Geometry check sheet. Reference: the model listing, model coordinates, mm. A direction names the side the tool comes from. Round coordinates to 2 decimals unless told otherwise and drop trailing zeros. Write each loop counter-clockwise with the first axis right and the second up, starting at its lowest first coordinate (ties: lowest second). Pieces come first, ordered by that corner, then holes. Notation, with made-up numbers: M 68,-39.5 L 116,-39.5 A20 cw 116,-7.5 Z; hole C -24.5,28.25 d3. An arc over 180 degrees is marked long. Answer in a Markdown table with one row per item. Add a question column.
from build123d import *

# Parameters (mm, degrees)
F3_DEPTH        = 5.5
F5_D            = 3.6
F5_COPIES_COUNT = 3
F6_SIZE         = 0.3


# Not quite as in the source:
# - a pattern or mirror of a feature is missing from the dataset's text; its kind, count and spacing are read off the source's solid


with BuildPart() as f1:
    # F0 (on Front) → F1 (revolve)
    with BuildSketch(Plane.XZ):
        Polygon((0, 11), (0, 0), (42, 0), (44.5, 2.5), (52.5, 2.5), (52.5, 3.5), (12, 3.5), (12, 2.5), (10, 2.5), (10, 3.5), (2, 3.5), (2, 11), align=None)
    revolve(axis=Axis((21, 0, 0), (-1, 0, 0)))

    # F2 (on face) → F3 (cut)
    with BuildSketch(Plane.YZ.offset(52.5)):
        with BuildLine():
            Line((2.5, 0), (3.5, 0))
            ThreePointArc((3.5, 0), (0, 3.5), (-3.5, 0))
            Line((-3.5, 0), (-2.5, 0))
            ThreePointArc((-2.5, 0), (0, 2.5), (2.5, 0))
        make_face()
    extrude(amount=-F3_DEPTH, mode=Mode.SUBTRACT)

    # F5 (through all)
    with Locations(Plane(origin=(0, 0, 0), x_dir=(0, -1, 0), z_dir=(-1, 0, 0))):
        with Locations((0, 7)):
            f5 = Hole(F5_D / 2)

    # F5_copies: F5 ×3 about axis
    f5_copies_axis = Axis((0, 0, 0), (1, 0, 0))
    for i in range(1, F5_COPIES_COUNT):
        add(f5.rotate(f5_copies_axis, i * 360 / F5_COPIES_COUNT), mode=Mode.SUBTRACT)

    # F6
    f6_edges = [f1.edges().sort_by_distance(p)[0] for p in [
        (0, 0, -11),
        (0, -6.962178, -1.941154),
        (0, 5.162178, -5.058846),
        (0, 1.8, 7),
    ]]
    chamfer(f6_edges, length=F6_SIZE)


solid = f1.part
Item 1: Access from +Z, -Z, +X, -X, +Y, -Y to the whole of each face (thin tool, end or side, straight path). Record for faces 4 (the cylindrical face through (31.966, 0.154, -3.497)), 5 (the flat face through (47, 0, 3)), 6 (the flat face through (12, -2, 2)), 7 (the cylindrical face through (1.162, -0.39, 5.243)), 8 (the flat face through (52.5, 0, -3)).
Item 2: Section check A-A, the plane x = 29. Record the boundary of the cut face in (y, z).
Item 3: Gauge pin test, flat ends, axial feed: pin 1 Ø3 at (y, z) = (-6.06, -3.5) entering from +X; pin 2 Ø4 at (x, z) = (13, -2.5) entering from +Y; pin 3 Ø0.8 at (x, y) = (51, 3) entering from +Z; pin 4 Ø8 at (x, z) = (45, -3.5) entering from -Y. Record the tip position at first contact, or that the pin passes through.
Item 4: Mould release check, pull along Y, two halves, no side actions. Record for faces 1 (the cylindrical face through (10.99, -2.44, -0.54)), 2 (the flat face through (50, -3, 0)), 3 (the cylindrical face through (1.162, 7.725, -4.189)): +Y half, -Y half, draft (parallel to the pull), parting line (faces both ways), or undercut.
Item 5: Section check B-B, the plane x = 48. Record the boundary of the cut face in (y, z), and give its area (3 significant figures).
Item 6: Scan lines: probe 1 along X at (y, z) = (-7.25, 3.75); probe 2 along Z at (x, y) = (46.5, 0); probe 3 along Z at (x, y) = (21.5, 3). Record each from-to range of solid material in increasing order. Write a range as from..to.
Result sheet:
| question | item | result |
|---|---|---|
| 1 | face 4 | +X |
| 1 | face 5 | +Z, +X, +Y, -Y |
| 1 | face 6 | none |
| 1 | face 7 | +X, -X |
| 1 | face 8 | +Z, -Z, +X, +Y, -Y |
| 2 | outline | C 0,0 d7 |
| 3 | pin 1 | passes through |
| 3 | pin 2 | stops at y = 3.46 |
| 3 | pin 3 | stops at z = 0 |
| 3 | pin 4 | stops at y = -3.5 |
| 4 | face 1 | parting line |
| 4 | face 2 | draft |
| 4 | face 3 | undercut |
| 5 | outline | M -3.5,0 A3.5 ccw 3.5,0 L 2.5,0 A2.5 cw -2.5,0 Z |
| 5 | area | 9.42 mm^2 |
| 6 | probe 1 | x = 0..2 |
| 6 | probe 2 | z = -3.5..-2.5, 2.5..3.5 |
| 6 | probe 3 | z = -1.8..1.8 |
